```python
from build123d import *

# Parameters (mm, degrees)
SKETCH2_W           = 54
SKETCH2_H           = 20
BOSS_EXTRUDE1_DEPTH = 2.5
SKETCH4_W           = 40.9
SKETCH4_H           = 20
BOSS_EXTRUDE2_DEPTH = 26.8
SKETCH5_W           = 40.9
SKETCH5_H           = 20
BOSS_EXTRUDE3_DEPTH = 7.7
SKETCH6_R           = 4
BOSS_EXTRUDE4_DEPTH = 5.7
SKETCH7_R           = 10
BOSS_EXTRUDE5_DEPTH = 2


with BuildPart() as part:
    # Sketch2 → Boss-Extrude1 (new body)
    with BuildSketch(Plane(origin=(0, 0, 0), x_dir=(1, 0, 0), z_dir=(0, 1, 0))):
        Rectangle(SKETCH2_W, SKETCH2_H)
    extrude(amount=BOSS_EXTRUDE1_DEPTH)

    # Sketch4 → Boss-Extrude2 (add)
    with BuildSketch(Plane.XZ):
        Rectangle(SKETCH4_W, SKETCH4_H)
    extrude(amount=BOSS_EXTRUDE2_DEPTH)

    # Sketch5 → Boss-Extrude3 (add)
    with BuildSketch(Plane(origin=(0, 2.5, 0), x_dir=(1, 0, 0), z_dir=(0, 1, 0))):
        Rectangle(SKETCH5_W, SKETCH5_H)
    extrude(amount=BOSS_EXTRUDE3_DEPTH)

    # Sketch6 → Boss-Extrude4 (add)
    with BuildSketch(Plane(origin=(0, 10.2, 0), x_dir=(1, 0, 0), z_dir=(0, 1, 0))):
        with Locations(Location((10.45, 0, 0), (0, 0, 90))):
            Circle(SKETCH6_R)
    extrude(amount=BOSS_EXTRUDE4_DEPTH)

    # Sketch7 → Boss-Extrude5 (add)
    with BuildSketch(Plane(origin=(0, 15.9, 0), x_dir=(1, 0, 0), z_dir=(0, 1, 0))):
        with Locations(Location((10.301103248, 0, 0), (0, 0, 270))):
            Circle(SKETCH7_R)
    extrude(amount=BOSS_EXTRUDE5_DEPTH)


solid = part.part
```
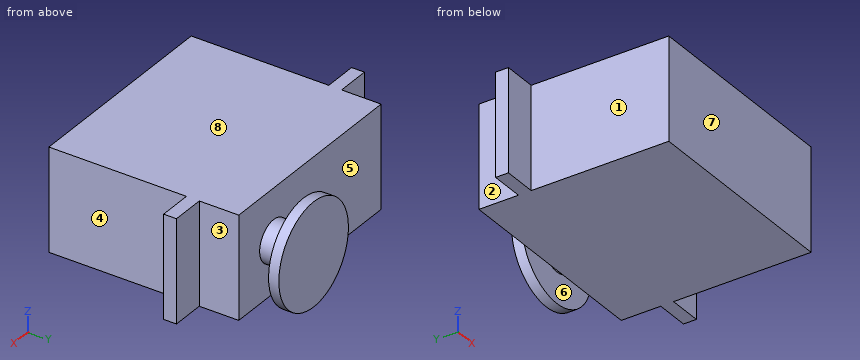
Work out the finished part from the listing and answer in its coordinate system (mm). Face numbers are marked on the shaded views. A direction names the side the tool comes from. Coordinates: 2 decimals unless noted, no trailing zeros. Write each loop counter-clockwise with the first axis right and the second up, starting at its lowest first coordinate (ties: lowest second). Pieces come first, ordered by that corner, then holes.
Q1. Each of these flat-tipped pins is pushed along its axis until it touches: pin 1 Ø12 at (x, z) = (-12.5, -0.5) entering from +Y; pin 2 Ø1 at (y, z) = (-14.5, -4.5) entering from +X; pin 3 Ø4 at (y, z) = (-20.5, 1.5) entering from -X. Where does it stop, or does it pass through?
Q2. Find the intervals of material crossed by line 1 (Y direction, x = 18.5, z = -2.5); line 2 (X direction, y = -12, z = -0.75); line 3 (Y direction, x = -9.5, z = 5.5), in increasing order.
Q3. A cutting plane is placed at B-B, the plane x = 4.5. Give the vertices of the cut face in (y, z).
Q4. Which of the six approach directions +Z, -Z, +X, -X, +Y, -Y give full straight-line access (tool end or side, diameter ignored) to the marked faces 1, 2, 3 and 4?
Q5. A cutting plane is placed at D-D, the plane y = -16. Give the vertices of the cut face in (x, z), then the cut area to 3 significant figures.
Q6. A cutting plane is placed at C-C, the plane z = -7.25. Give the vertices of the cut face in (x, y).
Q7. A cutting plane is placed at A-A, the plane z = 0. Give the vertices of the cut face in (x, y).
Q8. Determine the mould class of the marked faces 5, 6, 7 and 8 for opening direction Y: released by +Y, released by -Y, zero draft, split by the parting line, or undercut.
Findings below:
1. pin 1: stops at y = 10.2
1. pin 2: stops at x = 20.45
1. pin 3: stops at x = -20.45
2. line 1: y = -26.8 to 10.2, 15.9 to 17.9
2. line 2: x = -20.45 to 20.45
2. line 3: y = -26.8 to 10.2
3. outline: (-26.8, -10) - (10.2, -10) - (10.2, 10) - (-26.8, 10) - close; (15.9, -8.15) - (17.9, -8.15) - (17.9, 8.15) - (15.9, 8.15) - close
4. face 1: +Z, -Z, -X, -Y
4. face 2: +Z, -Z, -X, +Y
4. face 3: +Z, -Z, +X, +Y
4. face 4: +Z, -Z, +X, -Y
5. outline: (-20.45, -10) - (20.45, -10) - (20.45, 10) - (-20.45, 10) - close
5. area: 818 mm2
6. outline: (-27, 0) - (-20.45, 0) - (-20.45, -26.8) - (20.45, -26.8) - (20.45, 0) - (27, 0) - (27, 2.5) - (20.45, 2.5) - (20.45, 10.2) - (-20.45, 10.2) - (-20.45, 2.5) - (-27, 2.5) - close; (3.41, 15.9) - (17.19, 15.9) - (17.19, 17.9) - (3.41, 17.9) - close
7. outline: (-27, 0) - (-20.45, 0) - (-20.45, -26.8) - (20.45, -26.8) - (20.45, 0) - (27, 0) - (27, 2.5) - (20.45, 2.5) - (20.45, 10.2) - (14.45, 10.2) - (14.45, 15.9) - (20.3, 15.9) - (20.3, 17.9) - (0.3, 17.9) - (0.3, 15.9) - (6.45, 15.9) - (6.45, 10.2) - (-20.45, 10.2) - (-20.45, 2.5) - (-27, 2.5) - close
8. face 5: undercut
8. face 6: undercut
8. face 7: released by -Y
8. face 8: zero draft
